Read the model definition and answer for the solid it produces. Units are mm, in the model's axes. A direction names the side the tool comes from. Coordinates: 2 decimals unless noted, no trailing zeros. Loops run counter-clockwise (first coordinate to the right, second up) from the corner with the lowest first, then second, coordinate; pieces in that order, holes last.
Q1. Section C-C (z = -44.5) is taken. Give the vertices of the cut face in (x, y), then the cut area to 3 significant figures.
Q2. Flat-ended cylindrical pins translate along their axes: P1, Ø24, axis at x = 977.5, y = -54.5, coming from the -Z side; P2, Ø9, axis at x = 143, y = -164, coming from the -Z side; P3, Ø8, axis at x = 776, y = -220, coming from the +Z side. Find the tip coordinate at first contact, or state that the pin passes through.
Q3. Which of the six approach directions +Z, -Z, +X, -X, +Y, -Y give full straight-line access (tool end or side, diameter ignored) to faces 4 (the face through (965, -445, -248)), 5 (the face through (-945, -465, -248)), 6 (the face through (955, -2, 283)), 7 (the face through (13, -425, -49))?
Q4. Straight lines are drawn through the part: line 1 (X direction, y = 411.5, z = -61); line 2 (Y direction, x = -667, z = -35); line 3 (Z direction, x = 242.5, y = 431.5). For each, find the intervals that lie inside material, in ascending order.
Q5. Section D-D (y = -21.5) is taken. Count the separate pieces of the cut face and the enclosed holes in it, then the cut area to 4 significant figures.
Q6. Section B-B (z = 112.5) is taken. Give the vertices of the cut face in (x, y).
Q7. The mould has two halves that part along Y. Classify faces 1 (the face through (-13, 425, -49)), 2 (the face through (-965, 465, -400)), 3 (the face through (-151, 485, -78)): pulls with the +Y half, pulls with the -Y half, needs draft (parallel to the pull), parting line crosses it, or undercut.
Q8. Section A-A (x = -354) is taken. Give the vertices of the cut face in (y, z).
from build123d import *

# Parameters (mm, degrees)
F0_W     = 1970
F0_H     = 970
F0_W_2   = 30
F0_H_2   = 850
F1_DEPTH = 15
F2_DEPTH = 100
F3_W     = 30
F3_H     = 30
F3_W_2   = 20
F3_H_2   = 20
F4_DEPTH = 300
F5_W     = 30
F5_H     = 20
F6_DEPTH = 970
F7_W     = 40
F7_H     = 40
F8_DEPTH = 300


with BuildPart() as f1:
    # F0 (on Top) → F1 (new body)
    with BuildSketch(Plane.XY):
        Rectangle(F0_W, F0_H)
        Polygon((-925, -425), (-925, 425), (-880, 425), (-850, 425), (-802, 425), (-772, 425), (-724, 425), (-694, 425), (-646, 425), (-616, 425), (-568, 425), (-538, 425), (-490, 425), (-460, 425), (-412, 425), (-382, 425), (-334, 425), (-304, 425), (-256, 425), (-226, 425), (-178, 425), (-148, 425), (-100, 425), (-70, 425), (-22, 425), (8, 425), (56, 425), (86, 425), (134, 425), (164, 425), (212, 425), (242, 425), (290, 425), (320, 425), (368, 425), (398, 425), (446, 425), (476, 425), (524, 425), (554, 425), (602, 425), (632, 425), (680, 425), (710, 425), (758, 425), (788, 425), (836, 425), (866, 425), (925, 425), (925, -425), (866, -425), (836, -425), (788, -425), (758, -425), (710, -425), (680, -425), (632, -425), (602, -425), (554, -425), (524, -425), (476, -425), (446, -425), (398, -425), (368, -425), (320, -425), (290, -425), (242, -425), (212, -425), (164, -425), (134, -425), (86, -425), (56, -425), (8, -425), (-22, -425), (-70, -425), (-100, -425), (-148, -425), (-178, -425), (-226, -425), (-256, -425), (-304, -425), (-334, -425), (-382, -425), (-412, -425), (-460, -425), (-490, -425), (-538, -425), (-568, -425), (-616, -425), (-646, -425), (-694, -425), (-724, -425), (-772, -425), (-802, -425), (-850, -425), (-880, -425), align=None, mode=Mode.SUBTRACT)
        with Locations((-865, 0)):
            Rectangle(F0_W_2, F0_H_2)
        with Locations((-787, 0)):
            Rectangle(F0_W_2, F0_H_2)
        with Locations((-709, 0)):
            Rectangle(F0_W_2, F0_H_2)
        with Locations((-631, 0)):
            Rectangle(F0_W_2, F0_H_2)
        with Locations((-553, 0)):
            Rectangle(F0_W_2, F0_H_2)
        with Locations((-475, 0)):
            Rectangle(F0_W_2, F0_H_2)
        with Locations((-397, 0)):
            Rectangle(F0_W_2, F0_H_2)
        with Locations((-319, 0)):
            Rectangle(F0_W_2, F0_H_2)
        with Locations((-241, 0)):
            Rectangle(F0_W_2, F0_H_2)
        with Locations((-163, 0)):
            Rectangle(F0_W_2, F0_H_2)
        with Locations((-85, 0)):
            Rectangle(F0_W_2, F0_H_2)
        with Locations((-7, 0)):
            Rectangle(F0_W_2, F0_H_2)
        with Locations((71, 0)):
            Rectangle(F0_W_2, F0_H_2)
        with Locations((149, 0)):
            Rectangle(F0_W_2, F0_H_2)
        with Locations((227, 0)):
            Rectangle(F0_W_2, F0_H_2)
        with Locations((305, 0)):
            Rectangle(F0_W_2, F0_H_2)
        with Locations((383, 0)):
            Rectangle(F0_W_2, F0_H_2)
        with Locations((461, 0)):
            Rectangle(F0_W_2, F0_H_2)
        with Locations((539, 0)):
            Rectangle(F0_W_2, F0_H_2)
        with Locations((617, 0)):
            Rectangle(F0_W_2, F0_H_2)
        with Locations((695, 0)):
            Rectangle(F0_W_2, F0_H_2)
        with Locations((773, 0)):
            Rectangle(F0_W_2, F0_H_2)
        with Locations((851, 0)):
            Rectangle(F0_W_2, F0_H_2)
    extrude(amount=-F1_DEPTH)

    # F0 (on Top) → F2 (join)
    with BuildSketch(Plane.XY):
        Rectangle(F0_W, F0_H)
        Polygon((-925, -425), (-925, 425), (-880, 425), (-850, 425), (-802, 425), (-772, 425), (-724, 425), (-694, 425), (-646, 425), (-616, 425), (-568, 425), (-538, 425), (-490, 425), (-460, 425), (-412, 425), (-382, 425), (-334, 425), (-304, 425), (-256, 425), (-226, 425), (-178, 425), (-148, 425), (-100, 425), (-70, 425), (-22, 425), (8, 425), (56, 425), (86, 425), (134, 425), (164, 425), (212, 425), (242, 425), (290, 425), (320, 425), (368, 425), (398, 425), (446, 425), (476, 425), (524, 425), (554, 425), (602, 425), (632, 425), (680, 425), (710, 425), (758, 425), (788, 425), (836, 425), (866, 425), (925, 425), (925, -425), (866, -425), (836, -425), (788, -425), (758, -425), (710, -425), (680, -425), (632, -425), (602, -425), (554, -425), (524, -425), (476, -425), (446, -425), (398, -425), (368, -425), (320, -425), (290, -425), (242, -425), (212, -425), (164, -425), (134, -425), (86, -425), (56, -425), (8, -425), (-22, -425), (-70, -425), (-100, -425), (-148, -425), (-178, -425), (-226, -425), (-256, -425), (-304, -425), (-334, -425), (-382, -425), (-412, -425), (-460, -425), (-490, -425), (-538, -425), (-568, -425), (-616, -425), (-646, -425), (-694, -425), (-724, -425), (-772, -425), (-802, -425), (-850, -425), (-880, -425), align=None, mode=Mode.SUBTRACT)
    extrude(amount=-F2_DEPTH)

    # F3 (on face) → F4 (join)
    with BuildSketch(Plane.XY):
        with Locations((970, 470)):
            Rectangle(F3_W, F3_H)
        with Locations((970, -470)):
            Rectangle(F3_W, F3_H)
        with Locations((975, -80)):
            Rectangle(F3_W_2, F3_H_2)
        with Locations((975, 20)):
            Rectangle(F3_W_2, F3_H_2)
        with Locations((975, 120)):
            Rectangle(F3_W_2, F3_H_2)
    extrude(amount=F4_DEPTH)

    # F5 (on face) → F6 (join, through all)
    with BuildSketch(Plane.XZ.offset(485)):
        with Locations((970, 290)):
            Rectangle(F5_W, F5_H)
    extrude(amount=-F6_DEPTH)

    # F7 (on face) → F8 (join)
    with BuildSketch(Plane(origin=(0, 0, -100), x_dir=(1, 0, 0), z_dir=(0, 0, -1))):
        with Locations((965, 465)):
            Rectangle(F7_W, F7_H)
        with Locations((-965, 465)):
            Rectangle(F7_W, F7_H)
        with Locations((-965, -465)):
            Rectangle(F7_W, F7_H)
        with Locations((965, -465)):
            Rectangle(F7_W, F7_H)
    extrude(amount=F8_DEPTH)


solid = f1.part
Numbers:
1. outline: (-985, -485) - (985, -485) - (985, 485) - (-985, 485) - close; hole (-925, -425) - (925, -425) - (925, 425) - (-925, 425) - close
1. area: 338,000 mm2
2. P1: stops at z = -100
2. P2: stops at z = -15
2. P3: stops at z = 0
3. face 4: -Z, +X, -X
3. face 5: -Z, +Y, -Y
3. face 6: +Z, -X, +Y, -Y
3. face 7: -Z
4. line 1: x = -985 to -925, 925 to 985
4. line 2: y = -485 to -425, 425 to 485
4. line 3: z = -100 to 0
5. separate pieces: 26
5. enclosed holes: 0
5. area: 22,950 mm2
6. outline: (955, -485) - (985, -485) - (985, -455) - (955, -455) - close; (955, 455) - (985, 455) - (985, 485) - (955, 485) - close; (965, -90) - (985, -90) - (985, -70) - (965, -70) - close; (965, 10) - (985, 10) - (985, 30) - (965, 30) - close; (965, 110) - (985, 110) - (985, 130) - (965, 130) - close
7. face 1: undercut
7. face 2: needs draft
7. face 3: pulls with the +Y half
8. outline: (-485, -100) - (-425, -100) - (-425, 0) - (-485, 0) - close; (425, -100) - (485, -100) - (485, 0) - (425, 0) - close
